Answer from the drawing. Dimensions are ordinates in mm from the lowest x, y and z of the part. A direction names the side the tool comes from. Give positions to 0.01 mm unless a question says otherwise; leave off trailing zeros. Write each loop counter-clockwise with the first axis right and the second up, starting at its lowest first coordinate (ties: lowest second). Pieces come first, ordered by that corner, then holes.
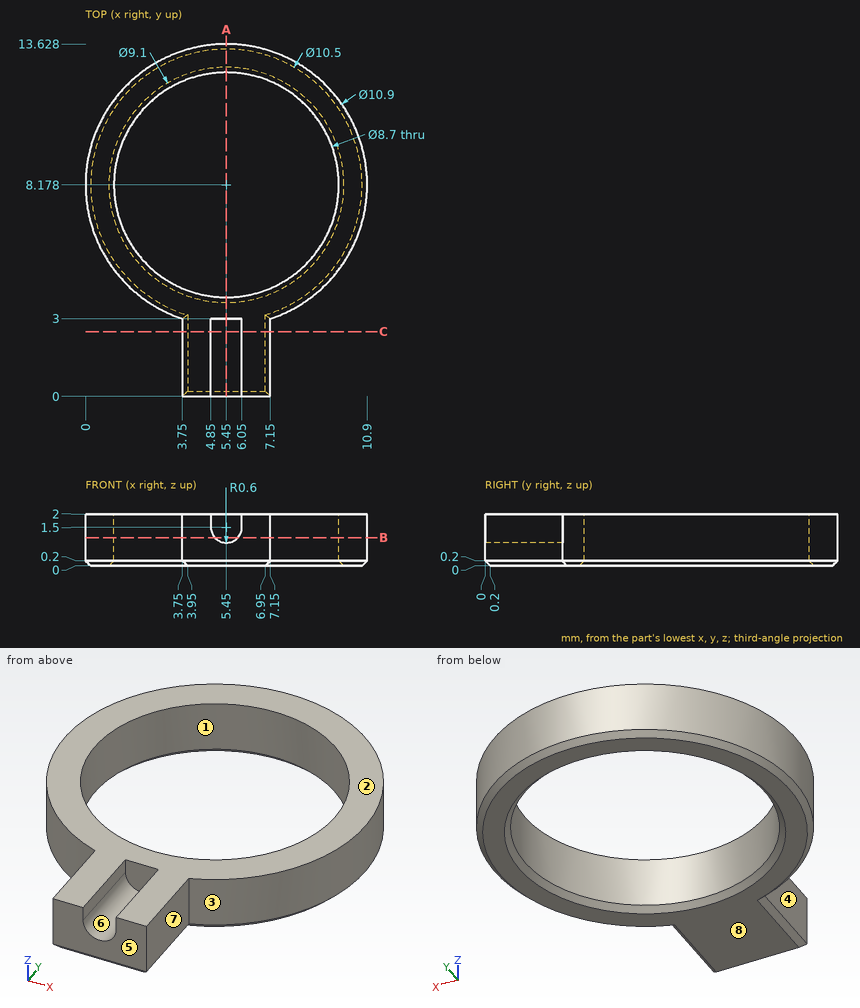
Item 1: Which of the six approach directions +Z, -Z, +X, -X, +Y, -Y give full straight-line access (tool end or side, diameter ignored) to the marked faces 4, 5, 6, 7 and 8?
Conclusion:
face 4: +Z, -Z, -X, -Y
face 5: +Z, -Z, +X, -X, -Y
face 6: +Z, -Y
face 7: +Z, -Z, +X, -Y
face 8: -Z, +X, -X, +Y, -Y
Item 2: A cutting plane is placed at A-A, the plane x = 5.45. Give the vertices of the cut face in (y, z).
Conclusion:
outline: (0, 0.2) - (0.2, 0) - (3.63, 0) - (3.83, 0.2) - (3.83, 2) - (3, 2) - (3, 0.9) - (0, 0.9) - close; (12.53, 0.2) - (12.73, 0) - (13.43, 0) - (13.63, 0.2) - (13.63, 2) - (12.53, 2) - close
Item 3: Determine the mould class of the marked faces 1, 2 and 3 for opening direction X: pulls with the +X half, pulls with the -X half, needs draft (parallel to the pull), parting line crosses it, or undercut.
Conclusion:
face 1: undercut
face 2: needs draft
face 3: parting line crosses it
Item 4: Consider probe 1 along X at (y, z) = (2.75, 1.85); probe 2 along Y at (x, z) = (5.45, 1.35); probe 3 along X at (y, z) = (7.5, 1.6). Determine where each line is inside the solid, lowest interval first.
Conclusion:
probe 1: x = 3.75 to 4.85, 6.05 to 7.15
probe 2: y = 3 to 3.83, 12.53 to 13.63
probe 3: x = 0.04 to 1.15, 9.75 to 10.86
Item 5: A cutting plane is placed at B-B, the plane z = 1.1. Give the vertices of the cut face in (x, y), plus the area to 3 significant figures.
Conclusion:
outline: (3.75, 0) - (5, 0) - (5, 3) - (5.9, 3) - (5.9, 0) - (7.15, 0) - (7.15, 3) arc R5.45 ccw (long way) to (3.75, 3) - close; hole circle Ø8.7 at (5.45, 8.18)
area: 40.8 mm2
Item 6: Each of these flat-tipped pins is pushed along its axis until it touches: P1, Ø0.5, axis at y = 1, z = 1.5, coming from the +X side; P2, Ø0.6, axis at x = 5.5, z = 1.5, coming from the -Y side; P3, Ø0.5, axis at y = 2, z = 1.5, coming from the -X side; P4, Ø1, axis at x = 4.5, y = 5, coming from the -Z side. Where does it stop, or does it pass through?
Conclusion:
P1: stops at x = 7.15
P2: stops at y = 3
P3: stops at x = 3.75
P4: passes through
Item 7: A cutting plane is placed at C-C, the plane y = 2.5. Give the vertices of the cut face in (x, z).
Conclusion:
outline: (3.75, 0.2) - (3.95, 0) - (6.95, 0) - (7.15, 0.2) - (7.15, 2) - (6.05, 2) - (6.05, 1.5) arc R0.6 cw to (4.85, 1.5) - (4.85, 2) - (3.75, 2) - close
